Design review of the part shown in the three views and the two pictorial views. Dimensions are in mm from the part's minimum x, y and z. Round coordinates to 2 decimals unless told otherwise and drop trailing zeros. Write each loop counter-clockwise with the first axis right and the second up, starting at its lowest first coordinate (ties: lowest second). Pieces come first, ordered by that corner, then holes. Notation, with made-up numbers: (6.5, -35) -> (18.5, -35) arc R19 cw to (18.5, -15) -> close; hole circle Ø3 at (86, 62). An arc over 180 degrees is marked (long way). Return JSON: item names as keys, results as strings. Group by question number.
1. Take a section at A-A, the plane z = 6.75. Write out the cut boundary in (x, y) (3 decimals), then the cut area to 3 significant figures.
2. Clearance check with a flat-ended pin moving along its axis: P1, Ø6.5, axis at x = 25.48, y = 25, coming from the +Z side. State where the tip first meets the part, or that it passes through.
3. Take a section at C-C, the plane y = 19.5. Write out the cut boundary in (x, z) (3 decimals), then the cut area to 3 significant figures.
4. Mouldability with a two-part tool opening along X and no side actions: class the marked faces 1, 2 and 3 as pulls with the +X half, pulls with the -X half, needs draft (parallel to the pull), parting line crosses it, or undercut.
5. Take a section at B-B, the plane y = 33. Write out the cut boundary in (x, z) (3 decimals), then the cut area to 3 significant figures.
6. For line 1 along X through (y, z) = (18.5, 6.25) (1 decimal); line 2 along Z through (x, y) = (29, 18); line 3 along Y through (x, z) = (23, 3), list the stretches that pass through material, from the lowest coordinate up. Write a range as from..to.
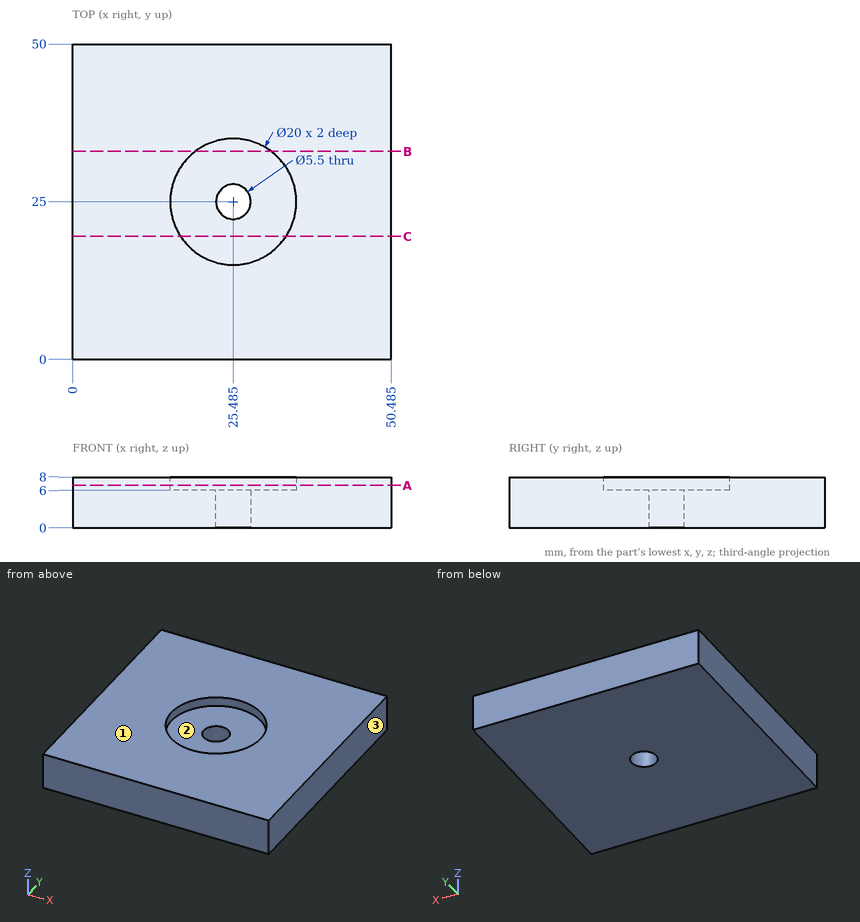
Output:
{
 "1": {"outline": "(0, 0) -> (50.485, 0) -> (50.485, 50) -> (0, 50) -> close; hole circle Ø20 at (25.485, 25)", "area": "2,210 mm^2"},
 "2": {"P1": "stops at z = 6"},
 "3": {"outline": "(0, 0) -> (50.485, 0) -> (50.485, 8) -> (33.837, 8) -> (33.837, 6) -> (17.133, 6) -> (17.133, 8) -> (0, 8) -> close", "area": "370 mm^2"},
 "4": {"face 1": "needs draft", "face 2": "undercut", "face 3": "pulls with the +X half"},
 "5": {"outline": "(0, 0) -> (50.485, 0) -> (50.485, 8) -> (31.485, 8) -> (31.485, 6) -> (19.485, 6) -> (19.485, 8) -> (0, 8) -> close", "area": "380 mm^2"},
 "6": {"line 1": "x = 0..17.9, 33.1..50.5", "line 2": "z = 0..6", "line 3": "y = 0..23.82, 26.18..50"}
}
